Autodesk Inventor part; units mm, degrees
ref_plane "YZ Plane" through (0, 0, 0) normal (1, 0, 0) x (0, 1, 0)
ref_plane "XZ Plane" through (0, 0, 0) normal (0, 1, 0) x (-1, 0, 0)
ref_plane "XY Plane" through (0, 0, 0) normal (0, 0, 1) x (1, 0, 0)
sketch "スケッチ1" plane through (0, 0, 0) normal (0, 1, 0) x (-1, 0, 0)
  circle A0 centre (0, 0) radius 8
  dimension "d0" = 16
extrude "押し出し1" add sketch "スケッチ1" along normal blind 70
sketch "スケッチ2" plane through (0, 70, 0) normal (0, 1, 0) x (1, 0, 0)
  circle A0 centre (0, 0) radius 8
sketch "スケッチ3" plane through (0, 70, 0) normal (0, 1, 0) x (1, 0, 0)
  circle A0 centre (0, 0) radius 8
  circle A1 centre (0, 0) radius 30
  dimension "d3" = 60
extrude "押し出し2" add sketch "スケッチ3" along normal blind 3
extrude "押し出し3" add sketch "スケッチ2" along normal blind 3
properties part number "知能ロボコン大砲４"
CAD build for the part. Positions are in the model's coordinates, mm. A direction names the side the tool comes from. Coordinates: 2 decimals unless noted, no trailing zeros. Write each loop counter-clockwise with the first axis right and the second up, starting at its lowest first coordinate (ties: lowest second). Pieces come first, ordered by that corner, then holes. Notation, with made-up numbers: (-24.75, -20.75) -> (-17.75, -20.75) arc R10 cw to (-17.75, -1.75) -> close; hole circle Ø4 at (51, 45). An arc over 180 degrees is marked (long way). Return JSON: item names as keys, results as strings. Group by question number.
Q1. Flat gauge pin, fed straight in: pin 1 (8 mm diameter, centred on y = 63.5, z = 10, fed in from -X). Where does the tip first touch, or does it go through?
Q2. Cut at D-D, the plane z = -13.5. Give the cut face in (x, y).
Q3. Cut at A-A, the plane z = 0. Give the cut face in (x, y), then the cut area to 3 significant figures.
Q4. Cut at B-B, the plane x = 0. Give the cut face in (y, z).
Q5. Cut at C-C, the plane y = 54.5. Give the cut face in (x, z).
Q6. Drill centre lines: line 1 (Y direction, x = -7, z = 6); line 2 (X direction, y = 62, z = -3.5); line 3 (X direction, y = 5.5, z = -4). Where is each one in solid material? Low to high.
Q7. Which spindle directions (+Z, -Z, +X, -X, +Y, -Y) get a long thin tool onto all of the face, cutting with end or side? Do faces 1 (the face through (1.73, 34.51, 7.81)), 2 (the face through (0, 0, 0)). Say none if no direction does.
Returned:
{
 "1": {"pin 1": "stops at x = -5.29"},
 "2": {"outline": "(-26.79, 70) -> (26.79, 70) -> (26.79, 73) -> (-26.79, 73) -> close"},
 "3": {"outline": "(-30, 70) -> (-8, 70) -> (-8, 0) -> (8, 0) -> (8, 70) -> (30, 70) -> (30, 73) -> (-30, 73) -> close", "area": "1,300 mm2"},
 "4": {"outline": "(0, -8) -> (70, -8) -> (70, -30) -> (73, -30) -> (73, 30) -> (70, 30) -> (70, 8) -> (0, 8) -> close"},
 "5": {"outline": "circle Ø16 at (0, 0)"},
 "6": {"line 1": "y = 70 to 73", "line 2": "x = -7.19 to 7.19", "line 3": "x = -6.93 to 6.93"},
 "7": {"face 1": "-Y", "face 2": "+Z, -Z, +X, -X, -Y"}
}
